Verification items for the finished model (mm, model axes). Face numbers are marked on the shaded views. A direction names the side the tool comes from. Give positions to 0.01 mm unless a question says otherwise; leave off trailing zeros. Write each loop counter-clockwise with the first axis right and the second up, starting at its lowest first coordinate (ties: lowest second). Pieces come first, ordered by that corner, then holes. Notation, with made-up numbers: (-3.5, 65) -> (12.5, 65) arc R18 cw to (12.5, 96) -> close; hole circle Ø6 at (10.5, -6). An arc over 180 degrees is marked (long way). Use one line per item in the form item = value. Start each with the question number.
(1) Section check C-C, the plane y = 38. Record the cut outline in (x, z), plus the area to 3 significant figures.
(2) Section check D-D, the plane y = -60.5. Record the cut outline in (x, z), plus the area to 3 significant figures.
(3) Depth check by flat-ended pin: pin 1 Ø10 at (x, y) = (103, -55.5) entering from +Z; pin 2 Ø10.5 at (y, z) = (-71.5, 75) entering from -X; pin 3 Ø24 at (x, y) = (16.5, -11.5) entering from +Z. Enter the tip coordinate at first touch or a pass-through.
(4) Release check for a two-part mould opening along X. For the marked faces 1, 2, 3 and 4 record: pulls with the +X half, pulls with the -X half, needs draft (parallel to the pull), parting line crosses it, or undercut.
(5) Section check B-B, the plane z = 17.5. Record the cut outline in (x, y), plus the area to 3 significant figures.
(6) Set-up check for the marked faces 5, 6 and 7: record each of +Z, -Z, +X, -X, +Y, -Y from which the full face is reachable in a straight line by a thin tool's end or side.
(7) Scan lines: L1, parallel to X at y = 27.5, z = 26; L2, parallel to X at y = -49, z = 60.5; L3, parallel to Y at x = 179, z = 17. Record each from-to range of solid material in increasing order.
(8) Section check A-A, the plane x = -113.5. Record the cut outline in (y, z).
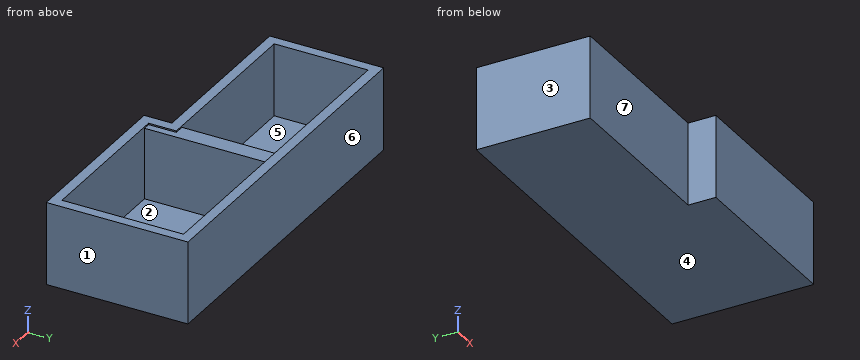
from build123d import *

# Parameters (mm, degrees)
F0_W     = 441.0978853703
F0_H     = 178.8222193718
F1_DEPTH = 104.1071284562
F2_W     = 220.5489426851
F2_H     = 34.9790751934
F3_DEPTH = 137.1856275946
F4_T     = -12.7
F5_W     = 21.9141840935
F5_H     = 178.8222193718
F6_DEPTH = 102.2892072797


with BuildPart() as f1:
    # F0 (on Top) → F1 (new body)
    with BuildSketch(Plane.XY):
        Rectangle(F0_W, F0_H)
    extrude(amount=F1_DEPTH)

    # F2 (on face) → F3 (cut)
    with BuildSketch(Plane.XY.offset(104.1071284562)):
        with Locations((-110.2744713426, -71.9215720892)):
            Rectangle(F2_W, F2_H)
    extrude(amount=-F3_DEPTH, mode=Mode.SUBTRACT)

    # F4
    f4_openings = [f1.faces().sort_by_distance(p)[0] for p in [
        (11.954487, 7.796778, 104.107128),
    ]]
    offset(amount=F4_T, openings=f4_openings, kind=Kind.INTERSECTION)

    # F5 (on face) → F6 (join)
    with BuildSketch(Plane(origin=(0, 0, 0), x_dir=(1, 0, 0), z_dir=(0, 0, -1))):
        with Locations((10.9570920467, 0)):
            Rectangle(F5_W, F5_H)
    extrude(amount=-F6_DEPTH)


solid = f1.part
Completed:
q1.outline = (-220.55, 0) -> (220.55, 0) -> (220.55, 104.11) -> (207.85, 104.11) -> (207.85, 12.7) -> (21.91, 12.7) -> (21.91, 102.29) -> (0, 102.29) -> (0, 12.7) -> (-207.85, 12.7) -> (-207.85, 104.11) -> (-220.55, 104.11) -> close
q1.area = 9,890 mm²
q2.outline = (0, 0) -> (220.55, 0) -> (220.55, 104.11) -> (207.85, 104.11) -> (207.85, 12.7) -> (21.91, 12.7) -> (21.91, 102.29) -> (12.7, 102.29) -> (12.7, 104.11) -> (0, 104.11) -> close
q2.area = 5,950 mm²
q3.pin_1 = 12.7
q3.pin_2 = 0
q3.pin_3 = 102.29
q4.face_1 = pulls with the +X half
q4.face_2 = undercut
q4.face_3 = pulls with the -X half
q4.face_4 = needs draft
q5.outline = (-220.55, -54.43) -> (0, -54.43) -> (0, -89.41) -> (220.55, -89.41) -> (220.55, 89.41) -> (-220.55, 89.41) -> close; hole (-207.85, -41.73) -> (0, -41.73) -> (0, 76.71) -> (-207.85, 76.71) -> close; hole (21.91, -76.71) -> (207.85, -76.71) -> (207.85, 76.71) -> (21.91, 76.71) -> close
q5.area = 18,000 mm²
q6.face_5 = +Z
q6.face_6 = +Z, -Z, +X, -X, +Y
q6.face_7 = +Z, -Z, -X, -Y
q7.L1 = -220.55 to -207.85, 0 to 21.91, 207.85 to 220.55
q7.L2 = -220.55 to 21.91, 207.85 to 220.55
q7.L3 = -89.41 to -76.71, 76.71 to 89.41
q8.outline = (-54.43, 0) -> (89.41, 0) -> (89.41, 104.11) -> (76.71, 104.11) -> (76.71, 12.7) -> (-41.73, 12.7) -> (-41.73, 104.11) -> (-54.43, 104.11) -> close
